Geometry check sheet. Reference: the model listing, model coordinates, mm. A direction names the side the tool comes from. Coordinates: 2 decimals unless noted, no trailing zeros. Order: outer loops, then holes, each group sorted by start corner. A loop starts at its lowest first (then second) coordinate and runs counter-clockwise, first axis right, second up. Notation, with made-up numbers: M 18,71 L 74,71 A29 cw 74,102 Z; hole C 40,20.5 d1. An arc over 180 degrees is marked long. One line per item, written item: value. Start each with the question number.
1) Draft check along X on faces 3 (the cylindrical face through (23, 4, 5)), 4 (the cylindrical face through (1, 3, 5)), 5 (the flat face through (19, 1, 5)), 6 (the flat face through (12, 5, 5)). Enter one of: pulls with the +X half, pulls with the -X half, needs draft (parallel to the pull), parting line crosses it, or undercut.
2) Go/stop test with flat-tipped pins: P1, Ø6, axis at x = 11, z = 8, coming from the -Y side; P2, Ø1, axis at y = 1, z = 7.5, coming from the +X side. Record where each tip stops, or that it passes through.
3) Access from +Z, -Z, +X, -X, +Y, -Y to the whole of each face (thin tool, end or side, straight path). Record for faces 1 (the flat face through (12, 2, 5)), 2 (the flat face through (13, 3, 0)).
4) Thickness scan on L1, parallel to Y at x = 6, z = 8.25; L2, parallel to X at y = 0.5, z = 5.5; L3, parallel to X at y = 1.95, z = 4.25. Record the ranges inside material, lowest first. Write a range as from..to.
5) Sectioned sample at B-B, the plane y = 1.75. Enter the section's corners in (x, z), then the cut area to 3 significant figures.
6) Sectioned sample at D-D, the plane y = 0.45. Enter the section's corners in (x, z).
7) Sectioned sample at C-C, the plane x = 14. Enter the section's corners in (y, z).
```python
from build123d import *

# Parameters (mm, degrees)
BOSS_EXTRUDE1_DEPTH = 10
FILLET2_R           = 5
FILLET3_R           = 5


with BuildPart() as part:
    # Sketch1 → Boss-Extrude1 (new body)
    with BuildSketch(Plane.XY):
        Polygon((0, 0), (0, 5), (25, 5), (25, 0), (19, 0), (19, 2), (5, 2), (5, 0), align=None)
    extrude(amount=BOSS_EXTRUDE1_DEPTH)

    # Fillet2
    fillet2_edges = [part.edges().sort_by_distance(p)[0] for p in [
        (0, 5, 5),
    ]]
    fillet(fillet2_edges, radius=FILLET2_R - 0.0001)  # a hair under: the kernel refuses the full size

    # Fillet3
    fillet3_edges = [part.edges().sort_by_distance(p)[0] for p in [
        (25, 5, 5),
    ]]
    fillet(fillet3_edges, radius=FILLET3_R - 0.0001)  # a hair under: the kernel refuses the full size


solid = part.part
```
Final values:
1. face 3: pulls with the +X half
1. face 4: pulls with the -X half
1. face 5: undercut
1. face 6: needs draft
2. P1: stops at y = 2
2. P2: stops at x = 24.97
3. face 1: +Z, -Z, -Y
3. face 2: -Z, +X, -X, +Y, -Y
4. L1: y = 2..5
4. L2: x = 0.03..5, 19..24.97
4. L3: x = 0.4..5, 19..24.6
5. outline: M 0.32,0 L 5,0 L 5,10 L 0.32,10 Z; M 19,0 L 24.68,0 L 24.68,10 L 19,10 Z
5. area: 104 mm^2
6. outline: M 0.02,0 L 5,0 L 5,10 L 0.02,10 Z; M 19,0 L 24.98,0 L 24.98,10 L 19,10 Z
7. outline: M 2,0 L 5,0 L 5,10 L 2,10 Z
